Could you check a few things on this model? Use its own coordinates, in mm. A direction names the side the tool comes from. Round coordinates to 2 decimals unless told otherwise and drop trailing zeros. Write each loop counter-clockwise with the first axis right and the second up, starting at its lowest first coordinate (ties: lowest second). Pieces come first, ordered by that corner, then holes. Notation, with made-up numbers: (54.25, 14.25) -> (100.25, 14.25) arc R17 cw to (100.25, 32.25) -> close; hole circle Ø7 at (-36.75, 53.25). An arc over 180 degrees is marked (long way). One line per question, with ' | ' between items. Start each with the question number.
1. Imagine slicing it at A-A, the plane z = 25. List the corners of the cut face in (x, y) for me.
2. If I drill on line 1 along X through (y, z) = (6.25, 26); line 2 along Y through (x, z) = (-3, 42.5); line 3 along X through (y, z) = (2, 43), over which ranges is the centre line in solid material (lowest first)? Write a range as [from, to].
3. Imagine slicing it at B-B, the plane y = 4. List the corners of the cut face in (x, z) for me, and give its area (3 significant figures).
4. For pin 1 Ø4 at (y, z) = (5, 16) entering from +X, with a flat end and sliding along its axis, tell me the tip position at first contact or that it passes through.
5. For faces 1 (the flat face through (1.8, 8, 24)), 2 (the flat face through (1.61, 0.785, 23.664)), 3 (the flat face through (-1.8, 8, 24)), which set-ups out of +Z, -Z, +X, -X, +Y, -Y let a thin tool reach every point of the face, with its end or its side?
6. Imagine slicing it at C-C, the plane x = -2.75. List the corners of the cut face in (y, z) for me, and give its area (3 significant figures).
from build123d import *

# Parameters (mm, degrees)
ESTRUSIONE_ESTRUSIONE1_DEPTH = 48


with BuildPart() as part:
    # Schizzo1 → Estrusione-Estrusione1 (new body)
    with BuildSketch(Plane.XY):
        with BuildLine():
            Line((0, 0), (-3.175204989, 1.548650948))
            ThreePointArc((-3.175204989, 1.548650948), (-3.287530759, 1.728409758), (-3.175204989, 1.908168567))
            Line((-3.175204989, 1.908168567), (-2.136976869, 2.414546255))
            ThreePointArc((-2.136976869, 2.414546255), (-1.891170699, 2.635871124), (-1.799999557, 2.953822683))
            Line((-1.799999557, 2.953822683), (-1.799999557, 12.578901072))
            Line((-1.799999557, 12.578901072), (1.799999557, 12.578901072))
            Line((1.799999557, 12.578901072), (1.799999557, 2.953822683))
            ThreePointArc((1.799999557, 2.953822683), (1.891170699, 2.635871124), (2.136976869, 2.414546255))
            Line((2.136976869, 2.414546255), (3.175204989, 1.908168567))
            ThreePointArc((3.175204989, 1.908168567), (3.287530759, 1.728409758), (3.175204989, 1.548650948))
            Line((3.175204989, 1.548650948), (0, 0))
        make_face()
    extrude(amount=ESTRUSIONE_ESTRUSIONE1_DEPTH)


solid = part.part
Geometry results:
1) outline: (-3.18, 1.55) -> (0, 0) -> (3.18, 1.55) arc R0.2 ccw to (3.18, 1.91) -> (2.14, 2.41) arc R0.6 cw to (1.8, 2.95) -> (1.8, 12.58) -> (-1.8, 12.58) -> (-1.8, 2.95) arc R0.6 cw to (-2.14, 2.41) -> (-3.18, 1.91) arc R0.2 ccw to start
2) line 1: x = [-1.8, 1.8] | line 2: y = [1.46, 1.99] | line 3: x = [-2.99, 2.99]
3) outline: (-1.8, 0) -> (1.8, 0) -> (1.8, 48) -> (-1.8, 48) -> close | area: 173 mm2
4) pin 1: stops at x = 1.8
5) face 1: +Z, -Z, +X, +Y | face 2: +Z, -Z, +X, -Y | face 3: +Z, -Z, -X, +Y
6) outline: (1.34, 0) -> (2.12, 0) -> (2.12, 48) -> (1.34, 48) -> close | area: 37.2 mm2
